Source: CAD feature listing. Evaluate the final solid. Frame: model axes, mm. Face numbers are marked on the shaded views. A direction names the side the tool comes from. Give positions to 0.01 mm unless a question says otherwise; leave off trailing zeros. Order: outer loops, then holes, each group sorted by start corner. A loop starts at its lowest first (then second) coordinate and runs counter-clockwise, first axis right, second up.
```python
from build123d import *

# Parameters (mm, degrees)
BOSS_EXTRUDE1_DEPTH = 3
BOSS_EXTRUDE2_DEPTH = 2


with BuildPart() as part:
    # Sketch1 → Boss-Extrude1 (new body)
    with BuildSketch(Plane(origin=(0, 0, 0), x_dir=(1, 0, 0), z_dir=(0, 1, 0))):
        Polygon((0, 4), (-3, 0), (3, 0), align=None)
    extrude(amount=BOSS_EXTRUDE1_DEPTH)

    # Sketch2 → Boss-Extrude2 (add)
    with BuildSketch(Plane(origin=(0, 3, 0), x_dir=(1, 0, 0), z_dir=(0, 1, 0))):
        Polygon((0, 0), (-3, 4), (3, 4), align=None)
    extrude(amount=BOSS_EXTRUDE2_DEPTH)


solid = part.part
```
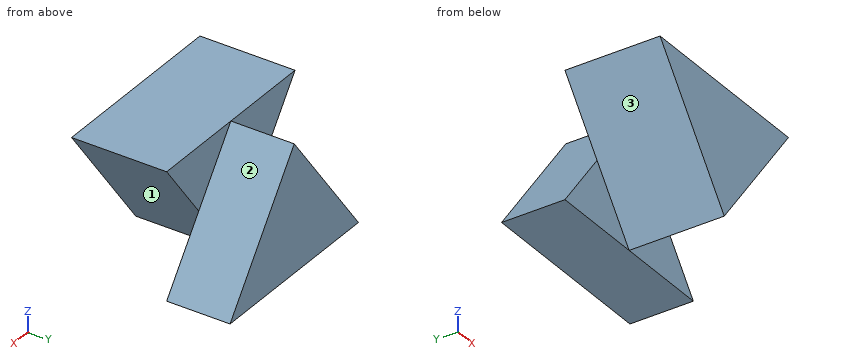
1) Reachability of the marked faces 1, 2 and 3 from +Z, -Z, +X, -X, +Y, -Y: full face, straight path, thin tool, end or side. Return the list, or none.
Report:
face 1: -Z, +X, -Y
face 2: +Z, +X, +Y
face 3: -Z, -X, -Y
2) Section query A-A, the plane z = -1.6. Return the cut outline in (x, y).
Report:
outline: (-1.8, 0) - (1.8, 0) - (1.8, 3) - (1.2, 3) - (1.2, 5) - (-1.2, 5) - (-1.2, 3) - (-1.8, 3) - close
3) Section query D-D, the plane y = 4.1. Return the cut outline in (x, z), and give its area (3 significant figures).
Report:
outline: (-3, -4) - (3, -4) - (0, 0) - close
area: 12.0 mm2
4) Pin query (flat end, axial travel): pin 1 (2 mm diameter, centred on x = -0.5, y = 4, fed in from +Z); pin 2 (0.6 mm diameter, centred on x = 1, z = -3.5, fed in from -Y). Return the tip coordinate at first contact, or that it passes through.
Report:
pin 1: stops at z = 0
pin 2: stops at y = 3
5) Material intervals for L1, parallel to Y at x = 2.1, z = -0.3; L2, parallel to Y at x = 1.5, z = -3.6; L3, parallel to X at y = 0.85, z = -2.6, sorted ascending.
Report:
L1: y = 0 to 3
L2: y = 3 to 5
L3: x = -1.05 to 1.05
6) Section query C-C, the plane x = 0.15. Return the cut outline in (y, z).
Report:
outline: (0, -3.8) - (3, -3.8) - (3, -4) - (5, -4) - (5, -0.2) - (3, -0.2) - (3, 0) - (0, 0) - close
7) Section query B-B, the plane x = 1.7. Return the cut outline in (y, z).
Report:
outline: (0, -1.73) - (3, -1.73) - (3, 0) - (0, 0) - close; (3, -4) - (5, -4) - (5, -2.27) - (3, -2.27) - close
